Geometry check sheet. Reference: the model listing, model coordinates, mm. A direction names the side the tool comes from. Round coordinates to 2 decimals unless told otherwise and drop trailing zeros. Order: outer loops, then holes, each group sorted by start corner. A loop starts at its lowest first (then second) coordinate and runs counter-clockwise, first axis right, second up.
(1) Thickness scan on L1, parallel to X at y = 2.9, z = 3; L2, parallel to Z at x = 3.5, y = 2.55 (3 decimals); L3, parallel to Z at x = 8.5, y = 1.55 (3 decimals). Record the ranges inside material, lowest first.
(2) Cross-section at A-A on y = 2.3. Count the separate pieces of the cut face and the enclosed holes in it, and give its area (3 significant figures).
(3) Cross-section at C-C on z = 6. Enter the section's corners in (x, y), and give its area (3 significant figures).
(4) Cross-section at B-B on x = 0. Enter the section's corners in (y, z) (3 decimals), and give its area (3 significant figures).
(5) Draft check along Z on faces 1 (the face through (0, 2, 27.045)), 2 (the face through (-19.97, 3.14, -25.54)), 3 (the face through (21.44, 2, 0)). Enter one of: pulls with the +Z half, pulls with the -Z half, needs draft (parallel to the pull), parting line crosses it, or undercut.
(6) Cross-section at D-D on x = -11.5. Enter the section's corners in (y, z) (3 decimals).
(7) Set-up check for faces 4 (the face through (-8.69, 2.26, 18.33)), 5 (the face through (-21.44, 2, 0)), 6 (the face through (-7.54, 1.77, 17.19)): record each of +Z, -Z, +X, -X, +Y, -Y from which the full face is reachable in a straight line by a thin tool's end or side.
from build123d import *

# Parameters (mm, degrees)
SKETCH1_W              = 11
SKETCH1_H              = 38.09
BOSS_EXTRUDE1_DEPTH    = 3
BOSS_EXTRUDE2_DEPTH    = 3
SKETCH3_W              = 40.88
SKETCH3_H              = 46.09
CUT_EXTRUDE1_DEPTH     = 2
MOVE_START             = 3
MOVE_FACE1_OUTLINE_W   = 42.88
MOVE_FACE1_OUTLINE_H   = 48.09
MOVE_FACE1_OUTLINE_W_2 = 40.88
MOVE_FACE1_OUTLINE_H_2 = 46.09
MOVE_FACE1_DEPTH       = 0.5
MOVE_FACE2_OUTLINE_W   = 18.88
MOVE_FACE2_OUTLINE_H   = 38.09
MOVE_FACE2_OUTLINE_W_2 = 16.88
MOVE_FACE2_OUTLINE_H_2 = 36.09
MOVE_FACE2_DEPTH       = 0.5
FILLET3_R              = 3
MOVE_FACE4_BY          = 3
MOVE_FACE5_BY          = 3
MOVE_FACE6_BY          = 3
MOVE_FACE7_BY          = 3
FILLET4_R              = 2.5
FILLET5_R              = 2
CHAMFER1_SIZE          = 0.5


# Read off the part's stored shape, not the designer's step: Move Face1, Move Face2
with BuildPart() as part:
    # Sketch1 → Boss-Extrude1 (new body)
    with BuildSketch(Plane(origin=(0, 0, 0), x_dir=(1, 0, 0), z_dir=(0, 1, 0))):
        Polygon((-9.44, 19.045), (0, 19.045), (9.44, 19.045), (9.44, -19.045), (20.44, -19.045), (20.44, 23.045), (-20.44, 23.045), (-20.44, 19.045), align=None)
        with Locations((-14.94, 0)):
            Rectangle(SKETCH1_W, SKETCH1_H)
        Polygon((9.44, -19.045), (0, -19.045), (-9.44, -19.045), (-20.44, -19.045), (-20.44, -23.045), (20.44, -23.045), (20.44, -19.045), align=None)
    extrude(amount=BOSS_EXTRUDE1_DEPTH)

    # Sketch2 → Boss-Extrude2 (add)
    with BuildSketch(Plane(origin=(0, 3, 0), x_dir=(1, 0, 0), z_dir=(0, 1, 0))):
        Polygon((20.44, 23.045), (20.44, -23.045), (21.44, -23.045), (21.44, 24.045), (-21.44, 24.045), (-21.44, 23.045), (-20.44, 23.045), align=None)
        Polygon((21.44, -23.045), (20.44, -23.045), (-20.44, -23.045), (-20.44, 23.045), (-21.44, 23.045), (-21.44, -24.045), (21.44, -24.045), align=None)
        Polygon((-8.44, 19.045), (-9.44, 19.045), (-9.44, -19.045), (8.44, -19.045), (8.44, -18.045), (-8.44, -18.045), (-8.44, 18.045), align=None)
        Polygon((9.44, 19.045), (-8.44, 19.045), (-8.44, 18.045), (8.44, 18.045), (8.44, -18.045), (8.44, -19.045), (9.44, -19.045), align=None)
    extrude(amount=-BOSS_EXTRUDE2_DEPTH)

    # Sketch3 → Cut-Extrude1 (cut)
    with BuildSketch(Plane(origin=(0, 3, 0), x_dir=(1, 0, 0), z_dir=(0, 1, 0))):
        Rectangle(SKETCH3_W, SKETCH3_H)
        Polygon((9.44, 19.045), (9.44, -18.045), (9.44, -19.045), (-9.44, -19.045), (-9.44, 18.045), (-9.44, 19.045), align=None, mode=Mode.SUBTRACT)
    extrude(amount=-CUT_EXTRUDE1_DEPTH, mode=Mode.SUBTRACT)

    # Move Face1 outline → Move Face1 (add)
    with BuildSketch(Plane(origin=(0, 0, 0), x_dir=(1, 0, 0), z_dir=(0, 1, 0)).offset(MOVE_START)):
        Rectangle(MOVE_FACE1_OUTLINE_W, MOVE_FACE1_OUTLINE_H)
        Rectangle(MOVE_FACE1_OUTLINE_W_2, MOVE_FACE1_OUTLINE_H_2, mode=Mode.SUBTRACT)
    extrude(amount=MOVE_FACE1_DEPTH)

    # Move Face2 outline → Move Face2 (add)
    with BuildSketch(Plane(origin=(0, 0, 0), x_dir=(1, 0, 0), z_dir=(0, 1, 0)).offset(MOVE_START)):
        Rectangle(MOVE_FACE2_OUTLINE_W, MOVE_FACE2_OUTLINE_H)
        Rectangle(MOVE_FACE2_OUTLINE_W_2, MOVE_FACE2_OUTLINE_H_2, mode=Mode.SUBTRACT)
    extrude(amount=MOVE_FACE2_DEPTH)

    # Fillet3
    fillet3_edges = [part.edges().sort_by_distance(p)[0] for p in [
        (-8.44, 1.75, -18.045),
        (-8.44, 1.75, 18.045),
        (8.44, 1.75, 18.045),
        (8.44, 1.75, -18.045),
    ]]
    fillet(fillet3_edges, radius=FILLET3_R)

    # Move Face4: a face moved outward by 3.0
    extrude(part.faces().sort_by_distance((0, 1.75, 24.045))[0], amount=MOVE_FACE4_BY, dir=(0, 0, 1))

    # Move Face5: a face moved outward by 3.0
    extrude(part.faces().sort_by_distance((0, 1.75, -24.045))[0], amount=MOVE_FACE5_BY, dir=(0, 0, -1))

    # Move Face6: a face moved inward by 3.0
    extrude(part.faces().sort_by_distance((0, 2.25, 23.045))[0], amount=MOVE_FACE6_BY, dir=(0, 0, 1), mode=Mode.SUBTRACT)

    # Move Face7: a face moved inward by 3.0
    extrude(part.faces().sort_by_distance((0, 2.25, -23.045))[0], amount=MOVE_FACE7_BY, dir=(0, 0, -1), mode=Mode.SUBTRACT)

    # Fillet4
    fillet4_edges = [part.edges().sort_by_distance(p)[0] for p in [
        (-9.44, 2.25, 19.045),
        (9.44, 2.25, 19.045),
        (9.44, 2.25, -19.045),
        (-9.44, 2.25, -19.045),
    ]]
    fillet(fillet4_edges, radius=FILLET4_R)

    # Fillet5
    fillet5_edges = [part.edges().sort_by_distance(p)[0] for p in [
        (-21.44, 1.75, 27.045),
        (-21.44, 1.75, -27.045),
        (21.44, 1.75, -27.045),
        (21.44, 1.75, 27.045),
        (-20.44, 2.25, 26.045),
        (-20.44, 2.25, -26.045),
        (20.44, 2.25, -26.045),
        (20.44, 2.25, 26.045),
    ]]
    fillet(fillet5_edges, radius=FILLET5_R)

    # Chamfer1
    chamfer1_edges = [part.edges().sort_by_distance(p)[0] for p in [
        (0, 3.5, 19.045),
        (0, 1, 19.045),
        (9.44, 3.5, 0),
        (0, 3.5, -19.045),
        (-9.44, 3.5, 0),
        (-8.707766953, 3.5, -18.312766953),
        (8.707766953, 3.5, -18.312766953),
        (-8.707766953, 3.5, 18.312766953),
        (8.707766953, 3.5, 18.312766953),
        (9.44, 1, 0),
        (-9.44, 1, 0),
        (0, 1, -19.045),
        (8.707766953, 1, 18.312766953),
        (-8.707766953, 1, 18.312766953),
        (8.707766953, 1, -18.312766953),
        (-8.707766953, 1, -18.312766953),
        (0, 3.5, -26.045),
        (0, 1, -26.045),
        (20.44, 3.5, 0),
        (20.44, 1, 0),
        (-20.44, 1, 0),
        (0, 1, 26.045),
        (19.854213562, 1, 25.459213562),
        (-19.854213562, 1, 25.459213562),
        (-19.854213562, 1, -25.459213562),
        (19.854213562, 1, -25.459213562),
        (-20.44, 3.5, 0),
        (0, 3.5, 26.045),
        (19.854213562, 3.5, -25.459213562),
        (-19.854213562, 3.5, -25.459213562),
        (-19.854213562, 3.5, 25.459213562),
        (19.854213562, 3.5, 25.459213562),
    ]]
    chamfer(chamfer1_edges, length=CHAMFER1_SIZE)


solid = part.part
Found:
1. L1: x = -21.44 to -20.44, -9.44 to -8.44, 8.44 to 9.44, 20.44 to 21.44
1. L2: z = -27.045 to -26.045, -19.045 to -18.045, 18.045 to 19.045, 26.045 to 27.045
1. L3: z = -27.045 to -26.045, -18.499 to 18.499, 26.045 to 27.045
2. separate pieces: 2
2. enclosed holes: 2
2. area: 302 mm2
3. outline: (-21.44, 0) - (-8.44, 0) - (-8.44, 3.5) - (-8.94, 3.5) - (-9.44, 3) - (-9.44, 1.5) - (-9.94, 1) - (-19.94, 1) - (-20.44, 1.5) - (-20.44, 3) - (-20.94, 3.5) - (-21.44, 3.5) - close; (8.44, 0) - (21.44, 0) - (21.44, 3.5) - (20.94, 3.5) - (20.44, 3) - (20.44, 1.5) - (19.94, 1) - (9.94, 1) - (9.44, 1.5) - (9.44, 3) - (8.94, 3.5) - (8.44, 3.5) - close
3. area: 36.0 mm2
4. outline: (0, -27.045) - (3.5, -27.045) - (3.5, -26.545) - (3, -26.045) - (1.5, -26.045) - (1, -25.545) - (1, -19.545) - (1.5, -19.045) - (3, -19.045) - (3.5, -18.545) - (3.5, -18.045) - (0, -18.045) - close; (0, 18.045) - (3.5, 18.045) - (3.5, 18.545) - (3, 19.045) - (1.5, 19.045) - (1, 19.545) - (1, 25.545) - (1.5, 26.045) - (3, 26.045) - (3.5, 26.545) - (3.5, 27.045) - (0, 27.045) - close
4. area: 28.0 mm2
5. face 1: pulls with the +Z half
5. face 2: undercut
5. face 3: needs draft
6. outline: (0, -27.045) - (3.5, -27.045) - (3.5, -26.545) - (3, -26.045) - (1.5, -26.045) - (1, -25.545) - (1, 25.545) - (1.5, 26.045) - (3, 26.045) - (3.5, 26.545) - (3.5, 27.045) - (0, 27.045) - close
7. face 4: +Y
7. face 5: +Z, -Z, -X, +Y, -Y
7. face 6: +Y, -Y
